from build123d import *

# Parameters (mm, degrees)
F1_DEPTH = 12.7
F3_D     = 12.3444
F4_R     = 7.62
F5_W     = 76.2
F5_H     = 77.0487710834
F6_DEPTH = 7.62
F7_R     = 7.62


# Not quite as in the source:
# - a feature names something its author has since deleted; it is built from what else it names


with BuildPart() as f1:
    # F0 (on Front) → F1 (new body)
    with BuildSketch(Plane.XZ):
        Polygon((-38.1, -38.1), (38.1, -38.1), (38.1, -30.48), (38.1, 38.1), (-38.1, 38.1), align=None)
    extrude(amount=F1_DEPTH)

    # F3 (through all)
    with Locations(Plane.XZ.offset(12.7)):
        with Locations((-29.1592, 29.1592), (-14.5796, 29.1592), (0, 29.1592), (14.5796, 29.1592), (29.1592, 29.1592), (29.1592, 14.5796), (29.1592, 0), (29.1592, -14.5796), (29.1592, -29.1592), (14.5796, -29.1592), (14.5796, -14.5796), (14.5796, 0), (14.5796, 14.5796), (0, 14.5796), (0, 0), (0, -14.5796), (0, -29.1592), (-14.5796, -29.1592), (-14.5796, -14.5796), (-14.5796, 0), (-14.5796, 14.5796), (-29.1592, 14.5796), (-29.1592, 0), (-29.1592, -14.5796), (-29.1592, -29.1592)):
            Hole(F3_D / 2)

    # F4
    f4_edges = [f1.edges().sort_by_distance(p)[0] for p in [
        (-38.1, -6.35, 38.1),
        (38.1, -6.35, 38.1),
        (38.1, -6.35, -38.1),
        (-38.1, -6.35, -38.1),
    ]]
    fillet(f4_edges, radius=F4_R)

    # F5 (on face) → F6 (join)
    with BuildSketch(Plane.XZ.offset(12.7)):
        Rectangle(F5_W, F5_H)
    extrude(amount=F6_DEPTH)

    # F7
    f7_edges = [f1.edges().sort_by_distance(p)[0] for p in [
        (-38.1, -16.51, 38.524386),
        (38.1, -16.51, 38.524386),
        (38.1, -16.51, -38.524386),
        (-38.1, -16.51, -38.524386),
    ]]
    fillet(f7_edges, radius=F7_R)


solid = f1.part
Input: part model. Units: mm. Frame: model coordinates. A direction names the side the tool comes from. Give positions to 0.01 mm unless a question says otherwise; leave off trailing zeros. Order: outer loops, then holes, each group sorted by start corner. A loop starts at its lowest first (then second) coordinate and runs counter-clockwise, first axis right, second up. Notation, with made-up numbers: M 44,38 L 60,38 A7 cw 60,47 Z; hole C 59.5,-28 d8. An arc over 180 degrees is marked long. Answer as a JSON object with one key per item and string values.
1. Cut plane A-A, the plane z = 0. Output: boundary loops of the cut face in (x, y), and give its area (3 significant figures).
Result sheet:
{"outline": "M -38.1,-20.32 L 38.1,-20.32 L 38.1,0 L 35.33,0 L 35.33,-12.7 L 22.99,-12.7 L 22.99,0 L 20.75,0 L 20.75,-12.7 L 8.41,-12.7 L 8.41,0 L 6.17,0 L 6.17,-12.7 L -6.17,-12.7 L -6.17,0 L -8.41,0 L -8.41,-12.7 L -20.75,-12.7 L -20.75,0 L -22.99,0 L -22.99,-12.7 L -35.33,-12.7 L -35.33,0 L -38.1,0 Z", "area": "765 mm²"}
2. Cut plane C-C, the plane y = -3.25. State how many separate pieces and enclosed holes the cut face has, and give its area (3 significant figures).
Result sheet:
{"separate pieces": "1", "enclosed holes": "25", "area": "2,760 mm²"}
3. Reachability of faces 4 (the flat face through (38.1, -10, 0)), 5 (the flat face through (0, -12.7, 0)) from +Z, -Z, +X, -X, +Y, -Y: full face, straight path, thin tool, end or side. Return the list, or none.
Result sheet:
{"face 4": "+Z, -Z, +X, +Y, -Y", "face 5": "+Y"}
4. Cut plane B-B, the plane x = 28.5. Output: boundary loops of the cut face in (y, z).
Result sheet:
{"outline": "M -20.32,-38.52 L -12.7,-38.52 L -12.7,-38.1 L 0,-38.1 L 0,-35.3 L -12.7,-35.3 L -12.7,-23.02 L 0,-23.02 L 0,-20.72 L -12.7,-20.72 L -12.7,-8.44 L 0,-8.44 L 0,-6.14 L -12.7,-6.14 L -12.7,6.14 L 0,6.14 L 0,8.44 L -12.7,8.44 L -12.7,20.72 L 0,20.72 L 0,23.02 L -12.7,23.02 L -12.7,35.3 L 0,35.3 L 0,38.1 L -12.7,38.1 L -12.7,38.52 L -20.32,38.52 Z"}
5. Cut plane D-D, the plane x = 0. Output: boundary loops of the cut face in (y, z).
Result sheet:
{"outline": "M -20.32,-38.52 L -12.7,-38.52 L -12.7,-38.1 L 0,-38.1 L 0,-35.33 L -12.7,-35.33 L -12.7,-22.99 L 0,-22.99 L 0,-20.75 L -12.7,-20.75 L -12.7,-8.41 L 0,-8.41 L 0,-6.17 L -12.7,-6.17 L -12.7,6.17 L 0,6.17 L 0,8.41 L -12.7,8.41 L -12.7,20.75 L 0,20.75 L 0,22.99 L -12.7,22.99 L -12.7,35.33 L 0,35.33 L 0,38.1 L -12.7,38.1 L -12.7,38.52 L -20.32,38.52 Z"}
6. Ray query, line 1 (Z direction, x = 0, y = -3.75); line 2 (X direction, y = -11.5, z = -10). Return the intervals inside material, ascending. Write a range as [from, to].
Result sheet:
{"line 1": "[-38.1, -35.33], [-22.99, -20.75], [-8.41, -6.17], [6.17, 8.41], [20.75, 22.99], [35.33, 38.1]", "line 2": "[-38.1, -33.3], [-25.02, -18.72], [-10.44, -4.14], [4.14, 10.44], [18.72, 25.02], [33.3, 38.1]"}
7. First-contact query: P1, Ø7.5, axis at x = 29.16, z = -14.58, coming from the +Y side; P2, Ø10, axis at x = -16, z = 16, coming from the +Y side; P3, Ø6, axis at x = -9.5, y = -8, coming from the +Z side. Flat tips, straight axial feed; report the tip coordinate or a pass-through.
Result sheet:
{"P1": "y = -12.7", "P2": "y = 0", "P3": "z = 38.1"}
8. Pull-direction query (X, two-part tool) for faces 1 (the flat face through (0, -16, 38.524)), 2 (the cylindrical face through (23.27, -6.26, -27.31)), 3 (the cylindrical face through (35.81, -16.56, 36.35)); classes: +X half, -X half, draft (parallel to the pull), parting line (faces both ways), or undercut.
Result sheet:
{"face 1": "draft", "face 2": "undercut", "face 3": "+X half"}
